Can you work these out from the model? Positions are in its coordinate system, mm. A direction names the side the tool comes from. Coordinates: 2 decimals unless noted, no trailing zeros. Order: outer loops, then holes, each group sorted by start corner. A loop starts at its lowest first (then second) coordinate and runs counter-clockwise, first axis right, second up. Notation, with made-up numbers: (54, 20) -> (90, 20) arc R31 cw to (90, 58) -> close; hole circle Ø8 at (45.25, 41). An arc over 180 degrees is marked (long way). Answer as CSV lines item,"result".
from build123d import *

# Parameters (mm, degrees)
SKETCH1_W             = 83
SKETCH1_H             = 50
BOSS_EXTRUDE1_DEPTH   = 3
SKETCH2_W             = 50
SKETCH2_H             = 7
BOSS_EXTRUDE2_DEPTH   = 3.5
SKETCH3_W             = 16.057447236
SKETCH3_H             = 12.6
SKETCH3_W_2           = 10
BOSS_EXTRUDE3_DEPTH   = 31.93
M3X0_5_TAPPED_HOLE1_D = 2.5
SKETCH6_W             = 58.057447236
SKETCH6_H             = 20
BOSS_EXTRUDE4_DEPTH   = 15.18
SKETCH10_W            = 32
SKETCH10_H            = 12
CUT_EXTRUDE2_DEPTH    = 15.18
CUT_EXTRUDE4_REACH    = 61.727
SKETCH12_W            = 10
SKETCH12_H            = 4.6
SKETCH13_W            = 12
SKETCH13_H            = 8
BOSS_EXTRUDE5_DEPTH   = 33
SKETCH14_W            = 18
SKETCH14_H            = 3
BOSS_EXTRUDE6_DEPTH   = 8.057447236
FILLET1_R             = 5
FILLET2_R             = 5
FILLET3_R             = 2.5
FILLET4_R             = 2.5
FILLET5_R             = 2.5
M3X0_5_TAPPED_HOLE2_D = 2.5
SKETCH9_R             = 3.5
CUT_EXTRUDE1_DEPTH    = 65.034877071
FILLET6_R             = 2.5
CUT_EXTRUDE3_DEPTH    = 66.582356534
FILLET7_R             = 2
M3X0_5_TAPPED_HOLE3_D = 2.5


with BuildPart() as part:
    # Sketch1 → Boss-Extrude1 (new body)
    with BuildSketch(Plane(origin=(0, 0, 0), x_dir=(1, 0, 0), z_dir=(0, 1, 0))):
        Rectangle(SKETCH1_W, SKETCH1_H)
    extrude(amount=BOSS_EXTRUDE1_DEPTH)

    # Sketch2 → Boss-Extrude2 (add)
    with BuildSketch(Plane(origin=(0, 3, 0), x_dir=(1, 0, 0), z_dir=(0, 1, 0))):
        with Locations((-16.5, 21.5)):
            Rectangle(SKETCH2_W, SKETCH2_H)
        with Locations((-16.5, -1.5)):
            Rectangle(SKETCH2_W, SKETCH2_H)
    extrude(amount=BOSS_EXTRUDE2_DEPTH)

    # Sketch3 → Boss-Extrude3 (add)
    with BuildSketch(Plane(origin=(0, 3, 0), x_dir=(1, 0, 0), z_dir=(0, 1, 0))):
        with Locations((33.471276382, -18.7)):
            Rectangle(SKETCH3_W, SKETCH3_H)
        with Locations((-11.557447236, -18.7)):
            Rectangle(SKETCH3_W_2, SKETCH3_H)
    extrude(amount=BOSS_EXTRUDE3_DEPTH)

    # M3x0.5 Tapped Hole1 (through all)
    with Locations(Plane(origin=(0, 0, 12.4), x_dir=(-1, 0, 0), z_dir=(0, 0, -1))):
        with Locations((-28.442552764, 30.03), (-28.442552764, 22.03), (9.557447236, 22.03), (9.557447236, 30.03)):
            Hole(M3X0_5_TAPPED_HOLE1_D / 2)

    # Sketch6 → Boss-Extrude4 (add)
    with BuildSketch(Plane(origin=(0, 3, 0), x_dir=(1, 0, 0), z_dir=(0, 1, 0))):
        with Locations((12.471276382, -15)):
            Rectangle(SKETCH6_W, SKETCH6_H)
    extrude(amount=BOSS_EXTRUDE4_DEPTH)

    # Sketch10 → Cut-Extrude2 (cut)
    with BuildSketch(Plane(origin=(0, 18.18, 0), x_dir=(1, 0, 0), z_dir=(0, 1, 0))):
        with Locations((9.442552764, -15)):
            Rectangle(SKETCH10_W, SKETCH10_H)
    extrude(amount=-CUT_EXTRUDE2_DEPTH, mode=Mode.SUBTRACT)

    # Cut-Extrude4: up to this face of the body (flat: up to its plane)
    cut_extrude4_end = Plane(part.part.faces().sort_by_distance((9.442552764, 18.18, 23))[0])
    # Sketch12 → Cut-Extrude4 (cut, up to the picked face)
    with BuildSketch(Plane(origin=(0, 34.93, 0), x_dir=(1, 0, 0), z_dir=(0, 1, 0)), mode=Mode.PRIVATE) as cut_extrude4_sk1:
        with Locations((-11.557447236, -22.7)):
            Rectangle(SKETCH12_W, SKETCH12_H)
    cut_extrude4_tool1 = split(extrude(cut_extrude4_sk1.sketch, amount=-CUT_EXTRUDE4_REACH, mode=Mode.PRIVATE), bisect_by=cut_extrude4_end, keep=Keep.BOTH, mode=Mode.PRIVATE)
    add(cut_extrude4_tool1.solids().sort_by(Axis((-11.557447, 34.93, 22.7), (0, -1, 0)))[0], mode=Mode.SUBTRACT)

    # Sketch13 → Boss-Extrude5 (add)
    with BuildSketch(Plane.ZY.offset(16.557447236)):
        with Locations((16.5, 4)):
            Rectangle(SKETCH13_W, SKETCH13_H)
    extrude(amount=BOSS_EXTRUDE5_DEPTH)

    # Sketch14 → Boss-Extrude6 (add)
    with BuildSketch(Plane.ZY.offset(41.5)):
        with Locations((16, 1.5)):
            Rectangle(SKETCH14_W, SKETCH14_H)
    extrude(amount=BOSS_EXTRUDE6_DEPTH)

    # Fillet1
    fillet1_edges = [part.edges().sort_by_distance(p)[0] for p in [
        (8.5, 4.75, 5),
        (41.5, 10.59, 5),
        (-16.557447236, 4.75, 5),
    ]]
    fillet(fillet1_edges, radius=FILLET1_R)

    # Fillet2
    fillet2_edges = [part.edges().sort_by_distance(p)[0] for p in [
        (-16.557447236, 12.34, 5),
        (41.5, 1.5, -25),
    ]]
    fillet(fillet2_edges, radius=FILLET2_R)

    # Fillet3
    fillet3_edges = [part.edges().sort_by_distance(p)[0] for p in [
        (8.5, 4.75, -18),
        (-41.5, 4.75, -18),
        (-41.5, 4.75, -2),
        (8.5, 4.75, -2),
        (8.5, 4.75, -25),
        (-41.5, 4.75, 5),
        (-41.5, 3.25, -25),
    ]]
    fillet(fillet3_edges, radius=FILLET3_R)

    # Fillet4
    fillet4_edges = [part.edges().sort_by_distance(p)[0] for p in [
        (41.5, 18.18, 11.2),
        (40.035533906, 18.18, 6.464466094),
        (12.471276382, 18.18, 5),
        (-15.092981142, 18.18, 6.464466094),
        (-16.557447236, 18.18, 11.2),
        (4.442552764, 18.18, 25),
    ]]
    fillet(fillet4_edges, radius=FILLET4_R)

    # Fillet5
    fillet5_edges = [part.edges().sort_by_distance(p)[0] for p in [
        (-16.557447236, 34.93, 16.4),
        (-16.557447236, 26.555, 20.4),
        (-11.557447236, 34.93, 20.4),
        (-16.557447236, 18.18, 21.45),
        (-16.557447236, 9.34, 25),
        (33.471276382, 34.93, 25),
        (33.471276382, 34.93, 12.4),
        (41.5, 25.305, 12.4),
        (41.5, 34.93, 18.7),
        (41.5, 17.465, 25),
        (-16.557447236, 17.447766953, 24.267766953),
    ]]
    fillet(fillet5_edges, radius=FILLET5_R - 0.0001)  # a hair under: the kernel refuses the full size

    # M3x0.5 Tapped Hole2 (through all)
    with Locations(Plane(origin=(0, 6.5, 0), x_dir=(1, 0, 0), z_dir=(0, 1, 0))):
        with Locations((-37.99546971, -1.433732), (-15.066268, -1.49546971), (-15.00453029, 21.433732), (-37.933732, 21.49546971)):
            Hole(M3X0_5_TAPPED_HOLE2_D / 2)

    # Sketch9 → Cut-Extrude1 (cut, through all)
    with BuildSketch(Plane(origin=(0, 3, 0), x_dir=(1, 0, 0), z_dir=(0, 1, 0))):
        with Locations(Location((-16.5, 10, 0), (0, 0, 270))):
            Circle(SKETCH9_R)
    extrude(amount=-CUT_EXTRUDE1_DEPTH, mode=Mode.SUBTRACT)

    # Fillet6
    fillet6_edges = [part.edges().sort_by_distance(p)[0] for p in [
        (-6.557447236, 3, 15),
        (9.442552764, 3, 21),
        (25.442552764, 3, 15),
        (9.442552764, 3, 9),
        (25.442552764, 10.59, 21),
        (25.442552764, 10.59, 9),
        (-6.557447236, 10.59, 21),
        (-6.557447236, 10.59, 9),
    ]]
    fillet(fillet6_edges, radius=FILLET6_R)

    # Sketch11 → Cut-Extrude3 (cut, through all)
    with BuildSketch(Plane.XZ):
        with BuildLine():
            Line((-17, -25), (-16, -25))
            ThreePointArc((-16, -25), (-16.5, -24.5), (-17, -25))
        make_face()
    extrude(amount=-CUT_EXTRUDE3_DEPTH, mode=Mode.SUBTRACT)

    # Fillet7
    fillet7_edges = [part.edges().sort_by_distance(p)[0] for p in [
        (-49.557447236, 1.5, 7),
        (-41.5, 1.5, 7),
        (-49.557447236, 1.5, 25),
    ]]
    fillet(fillet7_edges, radius=FILLET7_R)

    # M3x0.5 Tapped Hole3 (through all)
    with Locations(Plane(origin=(0, 0, 0), x_dir=(-1, 0, 0), z_dir=(0, -1, 0))):
        with Locations((1.5, 10), (31.5, 10)):
            Hole(M3X0_5_TAPPED_HOLE3_D / 2)


solid = part.part
Q1. Which directions (+Z, -Z, +X, -X, +Y, -Y) give clear straight access to the entire face, cutting with the end or side of a thin tool? Please do faces 4 (the cylindrical face through (-17.983, 4.774, 6.504)), 5 (the cylindrical face through (24.73, 3.75, 14.95)), 6 (the flat face through (32, 25, 12.4)), 7 (the flat face through (-46, 1, 7)), 8 (the cylindrical face through (10.05, 4.77, 3.62)).
Solution:
face 4,"-X, +Y"
face 5,"+Y"
face 6,"-Z, +X, -X, +Y"
face 7,"-Z, -X, +Y, -Y"
face 8,"-Z, +X, +Y"
Q2. We'd pull the mould along Y, two halves only. Please class faces 1 (the cylindrical face through (-15.806, 34.217, 15.112)), 2 (the cylindrical face through (29.02, 20.92, 18.79)), 3 (the cylindrical face through (40.07, 1.52, -23.5)): pulls with the +Y half, pulls with the -Y half, needs draft (parallel to the pull), parting line crosses it, or undercut.
Solution:
face 1,"pulls with the +Y half"
face 2,"undercut"
face 3,"needs draft"
Q3. Imagine slicing it at A-A (z = -10). List the corners of the cut face in (x, y) for me, and give its area (3 significant figures).
Solution:
outline,"(-41.5, 0) -> (-32.75, 0) -> (-32.75, 3) -> (-41.5, 3) -> close; (-30.25, 0) -> (-20, 0) -> (-20, 3) -> (-30.25, 3) -> close; (-13, 0) -> (-2.75, 0) -> (-2.75, 3) -> (-13, 3) -> close; (-0.25, 0) -> (41.5, 0) -> (41.5, 3) -> (-0.25, 3) -> close"
area,"213 mm2"
Q4. For P1, Ø3, axis at x = -15, z = -21.43, coming from the +Y side; P2, Ø3, axis at y = 7.5, z = 7.5, coming from the -X side; P3, Ø3.5, axis at x = 11, z = 16.5, coming from the +Y side; P4, Ø10, axis at x = -25, y = 25, coming from the -Z side (3 decimals), each with a flat end and sliding along its axis, tell me the tip position at first contact or that it passes through.
Solution:
P1,"y = 6.5"
P2,"x = -18.11"
P3,"y = 3"
P4,"through"
Q5. Imagine slicing it at C-C (x = -31.5). List the corners of the cut face in (y, z) for me.
Solution:
outline,"(0, -25) -> (6.5, -25) -> (6.5, -18) -> (3, -18) -> (3, -11.25) -> (0, -11.25) -> close; (0, -8.75) -> (3, -8.75) -> (3, -2) -> (6.5, -2) -> (6.5, 5) -> (3, 5) -> (3, 10.5) -> (8, 10.5) -> (8, 22.5) -> (3, 22.5) -> (3, 25) -> (0, 25) -> close"
Q6. Imagine slicing it at D-D (y = 13). List the corners of the cut face in (x, z) for me, and give its area (3 significant figures).
Solution:
outline,"(-16.56, 10) arc R5 ccw to (-11.56, 5) -> (36.5, 5) arc R5 ccw to (41.5, 10) -> (41.5, 22.5) arc R2.5 ccw to (39, 25) -> (-14.06, 25) arc R2.5 ccw to (-16.56, 22.5) -> close; hole (-6.56, 11.5) arc R2.5 ccw to (-4.06, 9) -> (22.94, 9) arc R2.5 ccw to (25.44, 11.5) -> (25.44, 18.5) arc R2.5 ccw to (22.94, 21) -> (-4.06, 21) arc R2.5 ccw to (-6.56, 18.5) -> close"
area,"769 mm2"
Q7. If I drill on line 1 (X direction, y = 0.85, z = -10); line 2 (Z direction, x = -18, y = 3.5); line 3 (Z direction, x = 20.5, y = 11.5), over which ranges is the centre line in solid material (lowest first)?
Solution:
line 1,"-41.5 to -32.75, -30.25 to -20, -13 to -2.75, -0.25 to 41.5"
line 2,"-25 to -18, -2 to 6.49, 10.5 to 22.5"
line 3,"5 to 9, 21 to 25"
Q8. Imagine slicing it at B-B (y = 22.03). List the corners of the cut face in (x, z) for me.
Solution:
outline,"(-16.56, 12.4) -> (-10.81, 12.4) -> (-10.81, 20.4) -> (-14.06, 20.4) arc R2.5 ccw to (-16.56, 17.9) -> close; (-8.31, 12.4) -> (-6.56, 12.4) -> (-6.56, 18.5) arc R2.5 cw to (-5.68, 20.4) -> (-8.31, 20.4) -> close; (25.44, 12.4) -> (27.19, 12.4) -> (27.19, 25) -> (25.44, 25) -> close; (29.69, 12.4) -> (39, 12.4) arc R2.5 ccw to (41.5, 14.9) -> (41.5, 22.5) arc R2.5 ccw to (39, 25) -> (29.69, 25) -> close"
